Here's how the part is built. I have some questions about the finished solid (model axes, mm). A direction names the side the tool comes from. Round coordinates to 2 decimals unless told otherwise and drop trailing zeros. Order: outer loops, then holes, each group sorted by start corner. A loop starts at its lowest first (then second) coordinate and runs counter-clockwise, first axis right, second up. Notation, with made-up numbers: (-10.75, -5) -> (43.25, -5) arc R22 cw to (43.25, 12) -> close; hole circle Ø8 at (-26.75, 30). An arc over 180 degrees is marked (long way). Use a Markdown table: item, result. Add a question column.
from build123d import *

# Parameters (mm, degrees)
ESQUISSE1_W             = 20
ESQUISSE1_H             = 30
BOSS_EXTRU_1_DEPTH      = 15
CONG_1_R                = 7
ESQUISSE2_W             = 10
ESQUISSE2_H             = 15
ENL_V_MAT_EXTRU_1_DEPTH = 18.5
CONG_2_R                = 3
CONG_3_R                = 1.5
CHANFREIN1_SIZE         = 4.5
CONG_4_R                = 1.5
ENL_V_MAT_EXTRU_2_DEPTH = 0.5
ENL_V_MAT_EXTRU_3_DEPTH = 0.5


with BuildPart() as part:
    # Esquisse1 → Boss.-Extru.1 (new body)
    with BuildSketch(Plane.XY):
        Rectangle(ESQUISSE1_W, ESQUISSE1_H)
    extrude(amount=BOSS_EXTRU_1_DEPTH)

    # Congé1
    cong_1_edges = [part.edges().sort_by_distance(p)[0] for p in [
        (0, 15, 0),
        (0, 15, 15),
    ]]
    fillet(cong_1_edges, radius=CONG_1_R)

    # Esquisse2 → Enlèv. mat.-Extru.1 (cut)
    with BuildSketch(Plane(origin=(0, 15, 0), x_dir=(1, 0, 0), z_dir=(0, 1, 0))):
        with Locations((0, -7.5)):
            Rectangle(ESQUISSE2_W, ESQUISSE2_H)
    extrude(amount=-ENL_V_MAT_EXTRU_1_DEPTH, mode=Mode.SUBTRACT)

    # Congé2
    cong_2_edges = [part.edges().sort_by_distance(p)[0] for p in [
        (5, -3.5, 7.5),
        (-5, -3.5, 7.5),
    ]]
    fillet(cong_2_edges, radius=CONG_2_R)

    # Congé3
    cong_3_edges = [part.edges().sort_by_distance(p)[0] for p in [
        (-5, 12.949747468, 12.949747468),
        (5, 12.949747468, 12.949747468),
        (5, 12.949747468, 2.050252532),
        (-5, 12.949747468, 2.050252532),
        (-5, 15, 7.5),
        (5, 15, 7.5),
        (0, -3.5, 0),
        (0, -3.5, 15),
        (-5, 3.75, 15),
        (-5, 3.75, 0),
        (5, 3.75, 0),
        (5, 3.75, 15),
        (-4.121320344, -2.621320344, 15),
        (-4.121320344, -2.621320344, 0),
        (4.121320344, -2.621320344, 0),
        (4.121320344, -2.621320344, 15),
    ]]
    fillet(cong_3_edges, radius=CONG_3_R)

    # Chanfrein1
    chanfrein1_edges = [part.edges().sort_by_distance(p)[0] for p in [
        (10, -15, 7.5),
        (-10, -15, 7.5),
    ]]
    chamfer(chanfrein1_edges, length=CHANFREIN1_SIZE)

    # Congé4
    cong_4_edges = [part.edges().sort_by_distance(p)[0] for p in [
        (10, -1.25, 0),
        (10, -1.25, 15),
        (10, -10.5, 7.5),
        (0, -15, 0),
        (-7.75, -12.75, 0),
        (7.75, -12.75, 0),
        (0, -15, 15),
        (-5.5, -15, 7.5),
        (5.5, -15, 7.5),
        (-7.75, -12.75, 15),
        (7.75, -12.75, 15),
        (-10, -10.5, 7.5),
        (-10, 15, 7.5),
        (10, 15, 7.5),
        (-10, -1.25, 0),
        (-10, -1.25, 15),
        (-10, 12.949747468, 12.949747468),
        (-10, 12.949747468, 2.050252532),
        (10, 12.949747468, 12.949747468),
        (10, 12.949747468, 2.050252532),
    ]]
    fillet(cong_4_edges, radius=CONG_4_R)

    # Esquisse3 → Enlèv. mat.-Extru.2 (cut)
    with BuildSketch(Plane.XY.offset(15)):
        Polygon((6.799705196, -7.645408133), (4.313330171, -7.645408133), (3.525434873, -9.2634614), (2.411418382, -6.034839284), (0.730170893, -11.971446212), (0, -7.035440736), (-0.380916703, -7.817706498), (-2.785361583, -7.817706498), (-3.403636623, -9.087420826), (-4.398752101, -6.20339544), (-5.840764794, -7.645408133), (-7.399157136, -7.645408133), (-7.399157136, -8.045408133), (-5.675079369, -8.045408133), (-4.568230072, -6.938558836), (-3.466779638, -10.130762237), (-2.535235756, -8.217706498), (-0.22946322, -8.217706498), (0.607203371, -13.873630222), (2.449002124, -7.370105128), (3.462291858, -10.306802811), (4.563455998, -8.045408133), (6.799705196, -8.045408133), align=None)
    extrude(amount=-ENL_V_MAT_EXTRU_2_DEPTH, mode=Mode.SUBTRACT)

    # Esquisse4 → Enlèv. mat.-Extru.3 (cut)
    with BuildSketch(Plane.ZY.offset(10)):
        with BuildLine():
            Line((9.241265037, 9.282942777), (8, 10.85264875))
            Line((8, 10.85264875), (6.758734963, 9.282942777))
            ThreePointArc((6.758734963, 9.282942777), (6.827029099, 8.109971877), (8, 8.04167774))
            ThreePointArc((8, 8.04167774), (9.172970901, 8.109971877), (9.241265037, 9.282942777))
        make_face()
    extrude(amount=-ENL_V_MAT_EXTRU_3_DEPTH, mode=Mode.SUBTRACT)


solid = part.part
(1) I want a section at B-B on x = 1.5. List the corners of the cut face in (y, z) for me.
(2) I'm going to push flat-ended pins straight in: P1, Ø5, axis at x = 4.5, y = -3, coming from the -Z side; P2, Ø0.9, axis at y = 9, z = 8.5, coming from the -X side; P3, Ø0.6, axis at x = -1.5, z = 15, coming from the -Y side; P4, Ø2, axis at x = -5.5, z = 11.5, coming from the +Y side. Where does each tip first touch, or does it pass through?
(3) On a 3-axis mill with a long thin cutter (end or side, diameter ignored), from which of +Z, -Z, +X, -X, +Y, -Y can I reach the whole of each face in a straight line? I mean faces 4 (the cylindrical face through (-9.754, 8.123, 6.814)), 5 (the flat face through (-2, -7, 15)), 6 (the cylindrical face through (4.1, -2.64, 7.42)), 7 (the flat face through (-5.13, -7.5, 14.75)), 8 (the cylindrical face through (0.07, -14.55, 0.43)). Say none if no direction works.
(4) Please list where these lines run through material, in increasing order: probe 1 along X at (y, z) = (12, 3); probe 2 along Y at (x, z) = (-1.25, 11); probe 3 along Z at (x, y) = (-6.5, -8). Write a range as from..to.
(5) If we mould it in two halves opening along Z, with no side actions, what happens to faces 1 (the cylindrical face through (-5.43, 14.55, 7.51)), 2 (the cylindrical face through (-9.75, 8.1, 9.16)), 3 (the cylindrical face through (-5.43, 3.81, 0.45))? For each: pulls with the +Z half, pulls with the -Z half, needs draft (parallel to the pull), parting line crosses it, or undercut.
(6) I want a section at A-A on y = 1.75. List the corners of the cut face in (x, z) for me.
Output:
| question | item | result |
|---|---|---|
| 1 | outline | (-15, 1.5) arc R1.5 ccw to (-13.5, 0) -> (-5, 0) arc R1.5 ccw to (-3.5, 1.5) -> (-3.5, 13.5) arc R1.5 ccw to (-5, 15) -> (-9.25, 15) -> (-9.25, 14.5) -> (-10.72, 14.5) -> (-10.72, 15) -> (-13.5, 15) arc R1.5 ccw to (-15, 13.5) -> close |
| 2 | P1 | z = 0 |
| 2 | P2 | x = -9.5 |
| 2 | P3 | y = -14.4 |
| 2 | P4 | y = 14.4 |
| 3 | face 4 | -X |
| 3 | face 5 | +Z, +X, -X, +Y, -Y |
| 3 | face 6 | +Z, -Z, +Y |
| 3 | face 7 | +Z |
| 3 | face 8 | -Z, +X, -X, -Y |
| 4 | probe 1 | -9.99..-5.01, 5.01..9.99 |
| 4 | probe 2 | -15..-3.5 |
| 4 | probe 3 | 0..14.5 |
| 5 | face 1 | needs draft |
| 5 | face 2 | undercut |
| 5 | face 3 | pulls with the -Z half |
| 6 | outline | (-10, 1.5) arc R1.5 ccw to (-8.5, 0) -> (-6.5, 0) arc R1.5 ccw to (-5, 1.5) -> (-5, 13.5) arc R1.5 ccw to (-6.5, 15) -> (-8.5, 15) arc R1.5 ccw to (-10, 13.5) -> close; (5, 1.5) arc R1.5 ccw to (6.5, 0) -> (8.5, 0) arc R1.5 ccw to (10, 1.5) -> (10, 13.5) arc R1.5 ccw to (8.5, 15) -> (6.5, 15) arc R1.5 ccw to (5, 13.5) -> close |
